from build123d import *

# Parameters (mm, degrees)
SKETCH_2_W             = 15
SKETCH_2_H             = 24
EXTRUDE_1_DEPTH        = 2.6
SKETCH_5_W             = 15
SKETCH_5_H             = 13.4
EXTRUDE_2_DEPTH        = 2.6
FILLET_1_R             = 4
HOLE_WIZARD_M3_3_D     = 3.6
HOLE_WIZARD_M3_3_DEPTH = 32.75
HOLE_WIZARD_M3_3_TIP   = 1.081549114
FILLET_2_R             = 3
FILLET_3_R             = 3
HOLE_WIZARD_M3_5_DEPTH = 2.6


# Read off the part's stored shape, not the designer's step: M3 间隙槽口5
with BuildPart() as part:
    # 草图2 → 凸台-拉伸1 (new body)
    with BuildSketch(Plane(origin=(0, 0, 0), x_dir=(1, 0, 0), z_dir=(0, 1, 0))):
        with Locations((0, 12)):
            Rectangle(SKETCH_2_W, SKETCH_2_H)
    extrude(amount=EXTRUDE_1_DEPTH)

    # 草图5 → 凸台-拉伸2 (add)
    with BuildSketch(Plane.XY):
        with Locations((0, 9.3)):
            Rectangle(SKETCH_5_W, SKETCH_5_H)
        Polygon((-22.5, 16), (-7.5, 16), (7.5, 16), (22.5, 16), (22.5, 26), (-22.5, 26), align=None)
    extrude(amount=-EXTRUDE_2_DEPTH)

    # 圆角1
    fillet_1_edges = [part.edges().sort_by_distance(p)[0] for p in [
        (-7.5, 1.3, -24),
        (7.5, 1.3, -24),
    ]]
    fillet(fillet_1_edges, radius=FILLET_1_R)

    # M3 间隙槽口3
    with Locations(Plane.XY):
        with Locations((-18.5, 21), (18.5, 21)):
            Hole(HOLE_WIZARD_M3_3_D / 2, depth=HOLE_WIZARD_M3_3_DEPTH)
            with Locations((0, 0, -(HOLE_WIZARD_M3_3_DEPTH + HOLE_WIZARD_M3_3_TIP / 2))):  # 118° drill point
                Cone(0, HOLE_WIZARD_M3_3_D / 2, HOLE_WIZARD_M3_3_TIP, mode=Mode.SUBTRACT)

    # 圆角2
    fillet_2_edges = [part.edges().sort_by_distance(p)[0] for p in [
        (-22.5, 16, -1.3),
        (-22.5, 26, -1.3),
        (22.5, 26, -1.3),
        (22.5, 16, -1.3),
    ]]
    fillet(fillet_2_edges, radius=FILLET_2_R)

    # 圆角3
    fillet_3_edges = [part.edges().sort_by_distance(p)[0] for p in [
        (0, 2.6, -2.6),
    ]]
    fillet(fillet_3_edges, radius=FILLET_3_R)

    # M3 间隙槽口5 outline → M3 间隙槽口5 (cut)
    with BuildSketch(Plane(origin=(0, 0, 0), x_dir=(1, 0, 0), z_dir=(0, 1, 0))):
        with BuildLine():
            ThreePointArc((2.3, 8.8), (4, 10.5), (2.3, 12.2))
            Line((2.3, 12.2), (-2.3, 12.2))
            ThreePointArc((-2.3, 12.2), (-4, 10.5), (-2.3, 8.8))
            Line((-2.3, 8.8), (2.3, 8.8))
        make_face()
        with BuildLine():
            Line((-2.3, 16.8), (2.3, 16.8))
            ThreePointArc((2.3, 16.8), (4, 18.5), (2.3, 20.2))
            Line((2.3, 20.2), (-2.3, 20.2))
            ThreePointArc((-2.3, 20.2), (-4, 18.5), (-2.3, 16.8))
        make_face()
    extrude(amount=HOLE_WIZARD_M3_5_DEPTH, mode=Mode.SUBTRACT)


solid = part.part
Work out the finished part from the listing and answer in its coordinate system (mm). A direction names the side the tool comes from. Coordinates: 2 decimals unless noted, no trailing zeros. Loops run counter-clockwise (first coordinate to the right, second up) from the corner with the lowest first, then second, coordinate; pieces in that order, holes last. Notation, with made-up numbers: (-9, 15) -> (10, 15) arc R19 ccw to (10, 41) -> close; hole circle Ø2 at (-13.5, 70.25). An arc over 180 degrees is marked (long way). Answer as CSV lines item,"result".
1) For faces 4 (the face through (-7.5, 2, -6)), 5 (the face through (21.6, 16.86, -1.32)), 6 (the face through (4, 1.3, -10.5)), 7 (the face through (0, 2.6, -15)), 8 (the face through (6.359, 1.318, -22.797)), determine the directions among +Z, -Z, +X, -X, +Y, -Y from which every point of the face is accessible in a straight line to the end or side of a thin tool.
A:
face 4,"+Z, -Z, -X, -Y"
face 5,"+Z, -Z, +X, -Y"
face 6,"+Y, -Y"
face 7,"-Z, +X, -X, +Y"
face 8,"-Z, +X, +Y, -Y"
2) Flat-ended cylindrical pins translate along their axes: pin 1 (8 mm diameter, centred on x = -14.5, z = -18.5, fed in from +Y); pin 2 (3 mm diameter, centred on x = 15, z = -1.5, fed in from -Y); pin 3 (3 mm diameter, centred on x = -4, y = 10, fed in from -Z); pin 4 (8 mm diameter, centred on y = 11.5, z = -6, fed in from +X). Find the tip coordinate at first contact, or state that the pin passes through.
A:
pin 1,"passes through"
pin 2,"stops at y = 16"
pin 3,"stops at z = -2.6"
pin 4,"stops at x = 7.5"
3) The part is cut by section B-B (z = -10.5). Give the vertices of the cut face in (x, y), and give its area (3 significant figures).
A:
outline,"(-7.5, 0) -> (-4, 0) -> (-4, 2.6) -> (-7.5, 2.6) -> close; (4, 0) -> (7.5, 0) -> (7.5, 2.6) -> (4, 2.6) -> close"
area,"18.2 mm²"
4) Straight lines are drawn through the part: probe 1 along Y at (x, z) = (-18.5, -1.95); probe 2 along Z at (x, y) = (9.5, 23.5); probe 3 along X at (y, z) = (5.25, -2). For each, find the intervals that lie inside material, in ascending order.
A:
probe 1,"y = 16 to 19.2, 22.8 to 26"
probe 2,"z = -2.6 to 0"
probe 3,"x = -7.5 to 7.5"
5) For a pull along Z with two mould halves and no side action, classify faces 1 (the face through (0, 1, -24)), 2 (the face through (-21.64, 25.1, -1.32)), 3 (the face through (-4, 1.3, -18.5)) as released by +Z, released by -Z, zero draft, split by the parting line, or undercut.
A:
face 1,"released by -Z"
face 2,"zero draft"
face 3,"undercut"
6) The part is cut by section A-A (x = -18.5). Give the vertices of the cut face in (y, z), and give its area (3 significant figures).
A:
outline,"(16, -2.6) -> (19.2, -2.6) -> (19.2, 0) -> (16, 0) -> close; (22.8, -2.6) -> (26, -2.6) -> (26, 0) -> (22.8, 0) -> close"
area,"16.6 mm²"
7) The part is cut by section D-D (y = 13.25). Give the vertices of the cut face in (x, z).
A:
outline,"(-7.5, -2.6) -> (7.5, -2.6) -> (7.5, 0) -> (-7.5, 0) -> close"
8) The part is cut by section C-C (x = -4.5). Give the vertices of the cut face in (y, z), and give its area (3 significant figures).
A:
outline,"(0, -23.87) -> (2.6, -23.87) -> (2.6, -5.6) arc R3 cw to (5.6, -2.6) -> (26, -2.6) -> (26, 0) -> (0, 0) -> close"
area,"125 mm²"
